```python
from build123d import *

# Parameters (mm, degrees)
BOSS_EXTRUDE1_DEPTH = 6.35
SKETCH2_R           = 1.27
CUT_EXTRUDE1_DEPTH  = 7.35
LPATTERN1_COUNT     = 6
LPATTERN1_PITCH     = 6.35
SKETCH4_R           = 1.27
CUT_EXTRUDE2_DEPTH  = 7.35
FILLET1_R           = 3.175


with BuildPart() as part:
    # Sketch1 → Boss-Extrude1 (new body)
    with BuildSketch(Plane.XY):
        Polygon((0, 0), (101.6, 3.175), (101.6, 12.7), (0, 15.875), align=None)
    extrude(amount=BOSS_EXTRUDE1_DEPTH)

    # Sketch2 → Cut-Extrude1 (cut, through all)
    with BuildSketch(Plane.XY.offset(6.35)):
        with Locations((98.425, 7.9375)):
            Circle(SKETCH2_R)
    cut_extrude1 = extrude(amount=-CUT_EXTRUDE1_DEPTH, mode=Mode.SUBTRACT)

    # LPattern1: Cut-Extrude1 ×6
    with Locations(*[(-i * LPATTERN1_PITCH, 0, 0) for i in range(1, LPATTERN1_COUNT)]):
        add(cut_extrude1, mode=Mode.SUBTRACT)

    # Sketch4 → Cut-Extrude2 (cut, through all)
    with BuildSketch(Plane.XY.offset(6.35)):
        with Locations((3.175, 7.9375)):
            Circle(SKETCH4_R)
        with Locations((39.6875, 7.9375)):
            Circle(SKETCH4_R)
    extrude(amount=-CUT_EXTRUDE2_DEPTH, mode=Mode.SUBTRACT)

    # Fillet1
    fillet1_edges = [part.edges().sort_by_distance(p)[0] for p in [
        (0, 15.875, 3.175),
        (101.6, 12.7, 3.175),
        (101.6, 3.175, 3.175),
        (0, 0, 3.175),
    ]]
    fillet(fillet1_edges, radius=FILLET1_R)


solid = part.part
```
The model under review builds one solid part; all positions refer to its coordinate system, in mm. Give positions to 0.01 mm unless a question says otherwise; leave off trailing zeros. Write each loop counter-clockwise with the first axis right and the second up, starting at its lowest first coordinate (ties: lowest second). Pieces come first, ordered by that corner, then holes. Notation, with made-up numbers: (-23.5, 70.25) -> (1.5, 70.25) arc R14 cw to (1.5, 94.25) -> close; hole circle Ø10 at (-4, -39.75). An arc over 180 degrees is marked (long way). Put each result on its own line as item: value.
(1) The part is to be moulded in two halves that separate along Y. For faces 1 (the flat face through (50, 8, 0)), 2 (the cylindrical face through (71.756, 7.993, 3.219)), 3 (the cylindrical face through (0.94, 14.854, 3.219)), say which applies: pulls with the +Y half, pulls with the -Y half, needs draft (parallel to the pull), parting line crosses it, or undercut.
Results are:
face 1: needs draft
face 2: undercut
face 3: pulls with the +Y half
(2) We need section C-C, the plane y = 14.5. Give the boundary of the cut face in (x, z).
Results are:
outline: (0.63, 0) -> (44, 0) -> (44, 6.35) -> (0.63, 6.35) -> close
(3) To check wall thickness, follow probe 1 along Y at (x, z) = (80, 2.25) (3 decimals); probe 2 along Y at (x, z) = (78.5, 2); probe 3 along Y at (x, z) = (5.5, 2). State the ranges of each line that lie inside material, in increasing order. Write a range as from..to.
Results are:
probe 1: 2.5..6.832, 9.043..13.375
probe 2: 2.45..7.02, 8.86..13.42
probe 3: 0.17..15.7
(4) We need section A-A, the plane z = 5. State how many separate pieces and enclosed holes the cut face has, and give its area (3 significant figures).
Results are:
separate pieces: 1
enclosed holes: 8
area: 1,240 mm²
(5) For pin 1 Ø1.5 at (x, z) = (17, 2) entering from +Y, flat-tipped, find the tip position at first contact; note if it passes through.
Results are:
pin 1: y = 15.37
(6) We need section B-B, the plane x = 47. Give the boundary of the cut face in (y, z), and give its area (3 significant figures).
Results are:
outline: (1.47, 0) -> (14.41, 0) -> (14.41, 6.35) -> (1.47, 6.35) -> close
area: 82.2 mm²
